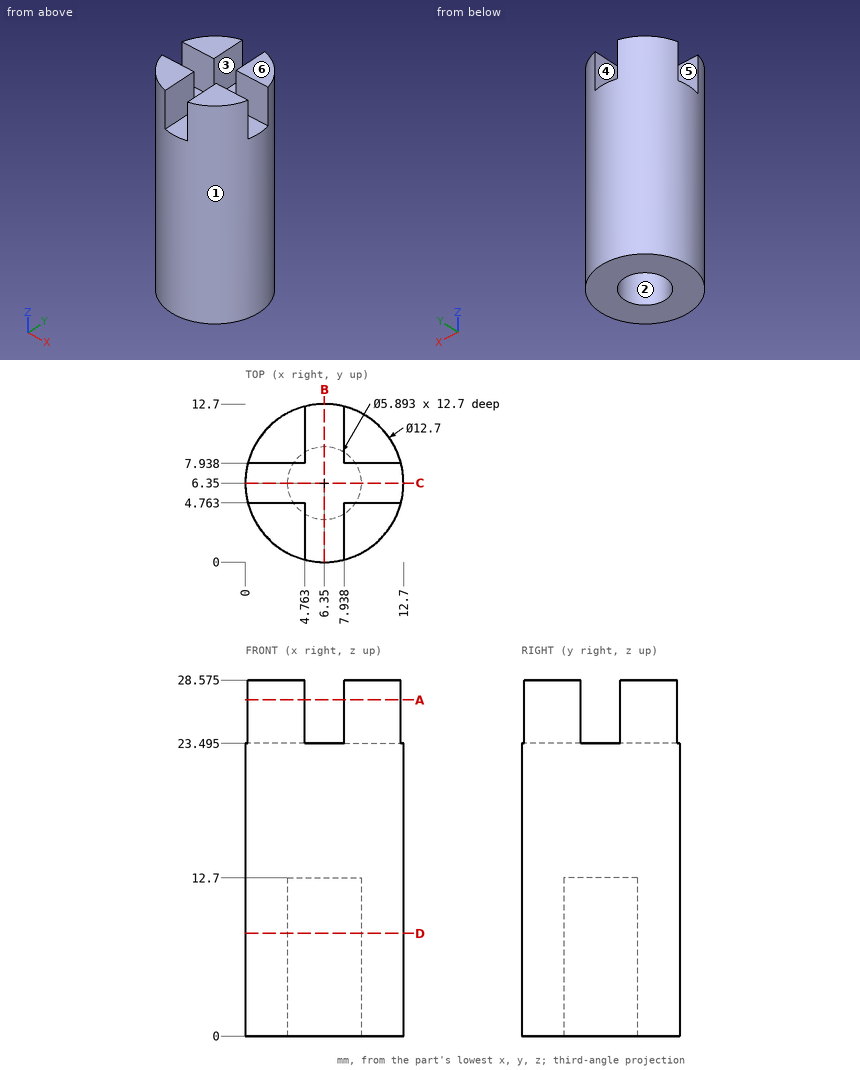
Design review of the part shown in the three views and the two pictorial views. Dimensions are in mm from the part's minimum x, y and z. A direction names the side the tool comes from. Coordinates: 2 decimals unless noted, no trailing zeros. Order: outer loops, then holes, each group sorted by start corner. A loop starts at its lowest first (then second) coordinate and runs counter-clockwise, first axis right, second up. Notation, with made-up numbers: (7, 3.25) -> (45, 3.25) arc R30 cw to (45, 33.25) -> close; hole circle Ø9 at (23.25, -22.5). An arc over 180 degrees is marked (long way). Use one line per item in the form item = value. Start each with the question number.
(1) For the marked faces 4, 5 and 6, list the 3-axis set-ups (+Z, -Z, +X, -X, +Y, -Y) from which the entire face can be reached by the end or side of a thin tool; tool diameter is ignored.
(2) The part is to be moulded in two halves that separate along Y. For the marked faces 1, 2 and 3, say which applies: +Y half, -Y half, draft (parallel to the pull), parting line (faces both ways), or undercut.
(3) Add section A-A on z = 27. State the section outline as (x, y) points.
(4) Add section B-B on x = 6.35. State the section outline as (y, z) points (1 decimal).
(5) Insertion check: pin 1 (1.4 mm diameter, centred on x = 9.5, z = 26, fed in from +Y); pin 2 (3.5 mm diameter, centred on x = 2.5, z = 26.5, fed in from +Y); pin 3 (1.5 mm diameter, centred on x = 2.5, z = 9.5, fed in from +Y). Each pin has a flat end and moves straight along its axis. Give the tip position at first contact, or say it passes through.
(6) For probe 1 along Y at (x, z) = (6.35, 6.5); probe 2 along X at (y, z) = (6.5, 3.5); probe 3 along Z at (x, y) = (5.5, 7.25) (1 decimal), list the stretches that pass through material, from the lowest coordinate up.
(7) Add section D-D on z = 8.25. State the section outline as (x, y) points.
Answer block:
q1.face_4 = +Z, +Y, -Y
q1.face_5 = +Z, +X, -X
q1.face_6 = +Z, +X, -X, +Y, -Y
q2.face_1 = parting line
q2.face_2 = undercut
q2.face_3 = draft
q3.outline = (0.2, 4.76) arc R6.35 ccw to (4.76, 0.2) -> (4.76, 4.76) -> close; (0.2, 7.94) -> (4.76, 7.94) -> (4.76, 12.5) arc R6.35 ccw to start; (7.94, 0.2) arc R6.35 ccw to (12.5, 4.76) -> (7.94, 4.76) -> close; (7.94, 7.94) -> (12.5, 7.94) arc R6.35 ccw to (7.94, 12.5) -> close
q4.outline = (0, 0) -> (3.4, 0) -> (3.4, 12.7) -> (9.3, 12.7) -> (9.3, 0) -> (12.7, 0) -> (12.7, 23.5) -> (0, 23.5) -> close
q5.pin_1 = 12.21
q5.pin_2 = 12.34
q5.pin_3 = 11.89
q6.probe_1 = 0 to 3.4, 9.3 to 12.7
q6.probe_2 = 0 to 3.41, 9.29 to 12.7
q6.probe_3 = 12.7 to 23.5
q7.outline = circle Ø12.7 at (6.35, 6.35); hole circle Ø5.89 at (6.35, 6.35)
